Verification items for the finished model (mm, model axes). Face numbers are marked on the shaded views. Round coordinates to 2 decimals unless told otherwise and drop trailing zeros. Write each loop counter-clockwise with the first axis right and the second up, starting at its lowest first coordinate (ties: lowest second). Pieces come first, ordered by that corner, then holes. Notation, with made-up numbers: M -8.75,-21.75 L 48.25,-21.75 A21 ccw 48.25,7.25 Z; hole C 84,43.25 d11. An arc over 180 degrees is marked long. One line per question, with ' | ' between items.
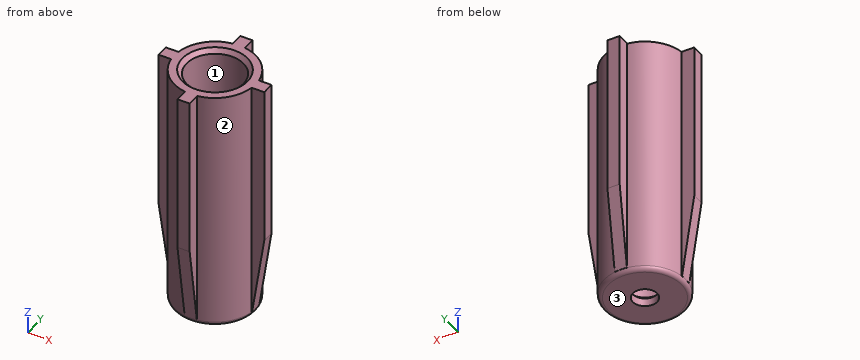
from build123d import *

# Parameters (mm, degrees)
F1_R        = 5
F1_R_2      = 3.5
F2_DEPTH    = 30
F4_W        = 1.5
F4_H        = 2.639524132
F5_DEPTH    = 29.5
F6_COUNT    = 4
F8_R        = 3.5
F8_R_2      = 1.5
F9_DEPTH    = 1.5
F10_SIZE2   = 1.49999
F10_SIZE    = 9.99999
F10_2_SIZE2 = 1.49999
F10_2_SIZE  = 9.99999
F10_3_SIZE2 = 1.49999
F10_3_SIZE  = 9.99999
F10_4_SIZE2 = 1.49999
F10_4_SIZE  = 9.99999
F11_SIZE    = 0.5
F12_R       = 0.49999


# Not quite as in the source:
# - a fillet or chamfer is up to 0.001 mm smaller than in the source, because OpenCascade refuses the exact size


with BuildPart() as f2:
    # F1 (on offset) → F2 (new body)
    with BuildSketch(Plane.XY):
        with Locations((-25, 25)):
            Circle(F1_R)
        with Locations((-25, 25)):
            Circle(F1_R_2, mode=Mode.SUBTRACT)
    extrude(amount=-F2_DEPTH)

    # F4 (on offset) → F5 (join)
    with BuildSketch(Plane.XY):
        with Locations((-25, 30.180237934)):
            Rectangle(F4_W, F4_H)
    extrude(amount=-F5_DEPTH)

    # F6: F2 ×4 about axis
    f6_axis = Axis((-25, 25, 0), (0, 0, 1))


with BuildPart() as f2_1:
    add(f2.part)
    for i in range(1, F6_COUNT):
        add(f2.part.rotate(f6_axis, i * 360 / F6_COUNT))

    # F8 (on offset) → F9 (join)
    with BuildSketch(Plane.XY.offset(-30)):
        with Locations((-25, 25)):
            Circle(F8_R)
        with Locations((-25, 25)):
            Circle(F8_R_2, mode=Mode.SUBTRACT)
    extrude(amount=F9_DEPTH)

    # F10 (size 10 and 1.5 in the source; OpenCascade refuses exactly that, so slightly less here)
    f10_edges = [f2_1.edges().sort_by_distance(p)[0] for p in [
        (-25, 18.5, -29.5),
    ]]
    f10_side = f2_1.faces().sort_by_distance((-25, 18.5, -14.75))[0]
    chamfer(f10_edges, length=F10_SIZE, length2=F10_SIZE2, reference=f10_side)

    # F10#2 (size 10 and 1.5 in the source; OpenCascade refuses exactly that, so slightly less here)
    f10_2_edges = [f2_1.edges().sort_by_distance(p)[0] for p in [
        (-18.5, 25, -29.5),
    ]]
    f10_2_side = f2_1.faces().sort_by_distance((-18.5, 25, -14.75))[0]
    chamfer(f10_2_edges, length=F10_2_SIZE, length2=F10_2_SIZE2, reference=f10_2_side)

    # F10#3 (size 10 and 1.5 in the source; OpenCascade refuses exactly that, so slightly less here)
    f10_3_edges = [f2_1.edges().sort_by_distance(p)[0] for p in [
        (-25, 31.5, -29.5),
    ]]
    f10_3_side = f2_1.faces().sort_by_distance((-25, 31.5, -14.75))[0]
    chamfer(f10_3_edges, length=F10_3_SIZE, length2=F10_3_SIZE2, reference=f10_3_side)

    # F10#4 (size 10 and 1.5 in the source; OpenCascade refuses exactly that, so slightly less here)
    f10_4_edges = [f2_1.edges().sort_by_distance(p)[0] for p in [
        (-31.5, 25, -29.5),
    ]]
    f10_4_side = f2_1.faces().sort_by_distance((-31.5, 25, -14.75))[0]
    chamfer(f10_4_edges, length=F10_4_SIZE, length2=F10_4_SIZE2, reference=f10_4_side)

    # F11
    f11_edges = [f2_1.edges().sort_by_distance(p)[0] for p in [
        (-28.5, 25, 0),
        (-26.5, 25, -28.5),
    ]]
    chamfer(f11_edges, length=F11_SIZE)

    # F12 (radius 0.5 in the source; OpenCascade refuses exactly that, so slightly less here)
    f12_edges = [f2_1.edges().sort_by_distance(p)[0] for p in [
        (-30, 25, -30),
    ]]
    fillet(f12_edges, radius=F12_R)


solid = f2_1.part
1. Mould release check, pull along Y, two halves, no side actions. Record for the marked faces 1, 2 and 3: pulls with the +Y half, pulls with the -Y half, needs draft (parallel to the pull), parting line crosses it, or undercut.
Results:
face 1: undercut | face 2: parting line crosses it | face 3: needs draft
2. Go/stop test with flat-tipped pins: P1, Ø0.5, axis at x = -31, z = -20.5, coming from the +Y side; P2, Ø1, axis at y = 29, z = -21, coming from the +X side; P3, Ø0.5, axis at y = 31, z = -18.5, coming from the +X side. Record where each tip stops, or that it passes through.
Results:
P1: stops at y = 25.75 | P2: stops at x = -21.43 | P3: stops at x = -24.25
3. Thickness scan on line 1 (X direction, y = 25, z = -8.25); line 2 (X direction, y = 30.25, z = -7.5); line 3 (Y direction, x = -25, z = -16). Record the ranges inside material, lowest first.
Results:
line 1: x = -31.5 to -28.5, -21.5 to -18.5 | line 2: x = -25.75 to -24.25 | line 3: y = 18.5 to 21.5, 28.5 to 31.5
4. Section check D-D, the plane z = -24.25. Record the cut outline in (x, y).
Results:
outline: M -30.79,24.25 L -29.94,24.25 A5 ccw -25.75,20.06 L -25.75,19.21 L -24.25,19.21 L -24.25,20.06 A5 ccw -20.06,24.25 L -19.21,24.25 L -19.21,25.75 L -20.06,25.75 A5 ccw -24.25,29.94 L -24.25,30.79 L -25.75,30.79 L -25.75,29.94 A5 ccw -29.94,25.75 L -30.79,25.75 Z; hole C -25,25 d7
5. Section check C-C, the plane z = -12. Record the cut outline in (x, y), then the cut area to 3 significant figures.
Results:
outline: M -31.5,24.25 L -29.94,24.25 A5 ccw -25.75,20.06 L -25.75,18.5 L -24.25,18.5 L -24.25,20.06 A5 ccw -20.06,24.25 L -18.5,24.25 L -18.5,25.75 L -20.06,25.75 A5 ccw -24.25,29.94 L -24.25,31.5 L -25.75,31.5 L -25.75,29.94 A5 ccw -29.94,25.75 L -31.5,25.75 Z; hole C -25,25 d7 | area: 49.2 mm2
